Build history of the part. All positions in model axes, mm. A direction names the side the tool comes from. Round coordinates to 2 decimals unless told otherwise and drop trailing zeros. Loops run counter-clockwise (first coordinate to the right, second up) from the corner with the lowest first, then second, coordinate; pieces in that order, holes last. Notation, with made-up numbers: (50.5, -29.5) - (58.5, -29.5) arc R30 cw to (58.5, -3.5) - close; hole circle Ø1 at (15, 38.5). An arc over 180 degrees is marked (long way). Use a Markdown table: item, result.
from build123d import *

# Parameters (mm, degrees)
CROQUIS1_R              = 7.5
SALIENTE_EXTRUIR1_DEPTH = 30
CROQUIS2_W              = 12
CROQUIS2_H              = 0.8
CORTAR_EXTRUIR1_DEPTH   = 37.193922142
CROQUIS3_R              = 1.05
CORTAR_EXTRUIR2_DEPTH   = 10
CROQUIS4_R              = 1.7
CORTAR_EXTRUIR3_DEPTH   = 41.902322672
CROQUIS5_R              = 2
CORTAR_EXTRUIR4_DEPTH   = 8


with BuildPart() as part:
    # Croquis1 → Saliente-Extruir1 (new body)
    with BuildSketch(Plane.XY):
        Polygon((-5, -11), (5, -11), (7.5, -7), (15.75, -7), (15.75, 3), (17, 5), (17, 10.4), (16.04, 11), (8.46, 11), (7.5, 10.4), (-7.5, 10.4), (-8.46, 11), (-16.04, 11), (-17, 10.4), (-17, 5), (-15.75, 3), (-15.75, -7), (-7.5, -7), align=None)
        Circle(CROQUIS1_R, mode=Mode.SUBTRACT)
    extrude(amount=SALIENTE_EXTRUIR1_DEPTH)

    # Croquis2 → Cortar-Extruir1 (cut, through all)
    with BuildSketch(Plane.XY.offset(30)):
        with Locations((11, -3.6)):
            Rectangle(CROQUIS2_W, CROQUIS2_H)
    extrude(amount=-CORTAR_EXTRUIR1_DEPTH, mode=Mode.SUBTRACT)

    # Croquis3 → Cortar-Extruir2 (cut)
    with BuildSketch(Plane.XZ.offset(7)):
        with Locations((11.625, 15)):
            Circle(CROQUIS3_R)
    extrude(amount=-CORTAR_EXTRUIR2_DEPTH, mode=Mode.SUBTRACT)

    # Croquis4 → Cortar-Extruir3 (cut, through all)
    with BuildSketch(Plane(origin=(0, 11, 0), x_dir=(1, 0, 0), z_dir=(0, 1, 0))):
        with Locations(Location((12, -6, 0), (0, 0, 180))):
            Circle(CROQUIS4_R)
        with Locations(Location((-12, -6, 0), (0, 0, 180))):
            Circle(CROQUIS4_R)
        with Locations(Location((-12, -24, 0), (0, 0, 180))):
            Circle(CROQUIS4_R)
        with Locations(Location((12, -24, 0), (0, 0, 180))):
            Circle(CROQUIS4_R)
    extrude(amount=-CORTAR_EXTRUIR3_DEPTH, mode=Mode.SUBTRACT)

    # Croquis5 → Cortar-Extruir4 (cut)
    with BuildSketch(Plane(origin=(0, 11, 0), x_dir=(1, 0, 0), z_dir=(0, 1, 0))):
        with Locations(Location((12, -6, 0), (0, 0, 180))):
            Circle(CROQUIS5_R)
        with Locations((-12, -6)):
            Circle(CROQUIS5_R)
        with Locations(Location((-12, -24, 0), (0, 0, 180))):
            Circle(CROQUIS5_R)
        with Locations((12, -24)):
            Circle(CROQUIS5_R)
    extrude(amount=-CORTAR_EXTRUIR4_DEPTH, mode=Mode.SUBTRACT)


solid = part.part
Q1. Pull direction Z, two halves, no side cores. Call faces 1 (the face through (4, 7, 0)), 2 (the face through (13.474, 7.056, 7.352)), 3 (the face through (12, 11, 15)): pulls with the +Z half, pulls with the -Z half, needs draft (parallel to the pull), parting line crosses it, or undercut.
Results found:
| item | result |
|---|---|
| face 1 | pulls with the -Z half |
| face 2 | undercut |
| face 3 | needs draft |
Q2. Probe line 1 (Z direction, x = -12, y = 6.75); line 2 (Z direction, x = 12, y = -4.6); line 3 (Y direction, x = 15.5, z = 26.75). List the from-to ranges inside material, lowest first.
Results found:
| item | result |
|---|---|
| line 1 | z = 0 to 4, 8 to 22, 26 to 30 |
| line 2 | z = 0 to 4.3, 7.7 to 14.02, 15.98 to 22.3, 25.7 to 30 |
| line 3 | y = -7 to -4, -3.2 to 11 |
Q3. Cut at D-D, the plane x = -12. List the corners of the cut face in (y, z), plus the area to 3 significant figures.
Results found:
| item | result |
|---|---|
| outline | (-7, 0) - (11, 0) - (11, 4) - (3, 4) - (3, 4.3) - (-7, 4.3) - close; (-7, 7.7) - (3, 7.7) - (3, 8) - (11, 8) - (11, 22) - (3, 22) - (3, 22.3) - (-7, 22.3) - close; (-7, 25.7) - (3, 25.7) - (3, 26) - (11, 26) - (11, 30) - (-7, 30) - close |
| area | 408 mm2 |
Q4. Cut at A-A, the plane x = 9. List the corners of the cut face in (y, z), plus the area to 3 significant figures.
Results found:
| item | result |
|---|---|
| outline | (-7, 0) - (-4, 0) - (-4, 30) - (-7, 30) - close; (-3.2, 0) - (11, 0) - (11, 30) - (-3.2, 30) - close |
| area | 516 mm2 |
Q5. Drop flat-ended pins along their axis: pin 1 (4.5 mm diameter, centred on x = 12, z = 6, fed in from +Y); pin 2 (5 mm diameter, centred on y = -7, z = 21, fed in from -X); pin 3 (5 mm diameter, centred on y = -7, z = 11.5, fed in from +X); pin 4 (0.6 mm diameter, centred on x = 11, z = 15, fed in from -Y). Give the stop position or say it passes through.
Results found:
| item | result |
|---|---|
| pin 1 | stops at y = 11 |
| pin 2 | stops at x = -15.75 |
| pin 3 | stops at x = 15.75 |
| pin 4 | stops at y = 3 |
Q6. Which spindle directions (+Z, -Z, +X, -X, +Y, -Y) get a long thin tool onto all of the face, cutting with end or side? Do faces 4 (the face through (-13.6, 7.1, 7.2)), 5 (the face through (12.11, -0.14, 14.07)), 6 (the face through (0, 10.4, 15)). Say none if no direction does.
Results found:
| item | result |
|---|---|
| face 4 | +Y |
| face 5 | -Y |
| face 6 | +Z, -Z, +Y |
Q7. Cut at B-B, the plane y = -1.75. List the corners of the cut face in (x, z) (3 decimals), plus the area to 3 significant figures.
Results found:
| item | result |
|---|---|
| outline | (-15.75, 0) - (-7.293, 0) - (-7.293, 30) - (-15.75, 30) - close; (7.293, 0) - (15.75, 0) - (15.75, 30) - (7.293, 30) - close; hole circle Ø3.4 at (-12, 6); hole circle Ø3.4 at (-12, 24); hole circle Ø3.4 at (12, 6); hole circle Ø3.4 at (12, 24); hole circle Ø2.1 at (11.625, 15) |
| area | 468 mm2 |
